```python
from build123d import *

# Parameters (mm, degrees)
SKETCH1_R           = 3.45
SKETCH1_R_2         = 7.5
SKETCH1_R_3         = 2.1
BOSS_EXTRUDE1_DEPTH = 1


with BuildPart() as part:
    # Sketch1 → Boss-Extrude1 (new body)
    with BuildSketch(Plane(origin=(0, 0, 0), x_dir=(1, 0, 0), z_dir=(0, 1, 0))):
        Polygon((-46, -80.5), (-61, -80.5), (-61, 80.5), (-46, 80.5), (-46, 95.5), (46, 95.5), (46, 80.5), (61, 80.5), (61, -80.5), (46, -80.5), (46, -95.5), (-46, -95.5), align=None)
        with Locations(Location((-34.8, 34.8, 0), (0, 0, 270))):
            Circle(SKETCH1_R, mode=Mode.SUBTRACT)
        with Locations(Location((34.8, 34.8, 0), (0, 0, 270))):
            Circle(SKETCH1_R, mode=Mode.SUBTRACT)
        with Locations(Location((34.8, -34.8, 0), (0, 0, 270))):
            Circle(SKETCH1_R, mode=Mode.SUBTRACT)
        with Locations(Location((-34.8, -34.8, 0), (0, 0, 270))):
            Circle(SKETCH1_R, mode=Mode.SUBTRACT)
        with Locations(Location((0, 0, 0), (0, 0, 270))):
            Circle(SKETCH1_R_2, mode=Mode.SUBTRACT)
        with Locations(Location((-43, -73, 0), (0, 0, 270))):
            Circle(SKETCH1_R_3, mode=Mode.SUBTRACT)
        with Locations(Location((43, -73, 0), (0, 0, 270))):
            Circle(SKETCH1_R_3, mode=Mode.SUBTRACT)
        with Locations(Location((-43, 73, 0), (0, 0, 270))):
            Circle(SKETCH1_R_3, mode=Mode.SUBTRACT)
        with Locations(Location((43, 73, 0), (0, 0, 270))):
            Circle(SKETCH1_R_3, mode=Mode.SUBTRACT)
    extrude(amount=BOSS_EXTRUDE1_DEPTH)


solid = part.part
```
Check sheet for the modelled part. Datum: model origin and axes. Units: mm. Round coordinates to 2 decimals unless told otherwise and drop trailing zeros. Loops run counter-clockwise (first coordinate to the right, second up) from the corner with the lowest first, then second, coordinate; pieces in that order, holes last. Notation, with made-up numbers: (41.25, 15.5) - (52.25, 15.5) arc R18 ccw to (52.25, 43.5) - close; hole circle Ø6 at (81, -13.5). An arc over 180 degrees is marked (long way). Write item = value, one per line. Start each with the question number.
Q1. Release check for a two-part mould opening along X. For faces 1 (the face through (38.22, 0.49, -35.25)), 2 (the face through (-32.468, 0.493, -37.343)), 3 (the face through (-13, 0, -1)) record: pulls with the +X half, pulls with the -X half, needs draft (parallel to the pull), parting line crosses it, or undercut.
Q2. Section check D-D (y = 0.45). Count the separate pieces of the cut face and the enclosed holes in it, plus the area to 3 significant figures.
Q3. Depth check by flat-ended pin: P1, Ø0.5, axis at x = -55.5, y = 0.5, coming from the -Z side; P2, Ø0.5, axis at y = 0.5, z = 90.5, coming from the -X side. Enter the tip coordinate at first touch or a pass-through.
Q4. Section check C-C (z = 0). Record the boundary of the cut face in (x, y).
Q5. Section check A-A (z = 34.8). Record the boundary of the cut face in (x, y), plus the area to 3 significant figures.
Q6. Thickness scan on L1, parallel to X at y = 0.35, z = 73; L2, parallel to X at y = 0.6, z = 34.8; L3, parallel to Z at x = -0.5, y = 0.35. Record the ranges inside material, lowest first.
Q7. Section check B-B (x = -34.8). Record the boundary of the cut face in (y, z).
Derived:
q1.face_1 = undercut
q1.face_2 = undercut
q1.face_3 = needs draft
q2.separate_pieces = 1
q2.enclosed_holes = 9
q2.area = 22,000 mm^2
q3.P1 = -80.5
q3.P2 = -46
q4.outline = (-61, 0) - (-7.5, 0) - (-7.5, 1) - (-61, 1) - close; (7.5, 0) - (61, 0) - (61, 1) - (7.5, 1) - close
q5.outline = (-61, 0) - (-38.25, 0) - (-38.25, 1) - (-61, 1) - close; (-31.35, 0) - (31.35, 0) - (31.35, 1) - (-31.35, 1) - close; (38.25, 0) - (61, 0) - (61, 1) - (38.25, 1) - close
q5.area = 108 mm^2
q6.L1 = -61 to -45.1, -40.9 to 40.9, 45.1 to 61
q6.L2 = -61 to -38.25, -31.35 to 31.35, 38.25 to 61
q6.L3 = -95.5 to -7.48, 7.48 to 95.5
q7.outline = (0, -95.5) - (1, -95.5) - (1, -38.25) - (0, -38.25) - close; (0, -31.35) - (1, -31.35) - (1, 31.35) - (0, 31.35) - close; (0, 38.25) - (1, 38.25) - (1, 95.5) - (0, 95.5) - close
